Source: CAD feature listing. Evaluate the final solid. Frame: model axes, mm. Face numbers are marked on the shaded views. A direction names the side the tool comes from. Give positions to 0.01 mm unless a question says otherwise; leave off trailing zeros. Order: outer loops, then holes, each group sorted by start corner. A loop starts at its lowest first (then second) coordinate and runs counter-clockwise, first axis right, second up. Notation, with made-up numbers: M 37,-27 L 57,-27 A24 ccw 57,1 Z; hole C -12.75,-10.75 d11. An arc over 180 degrees is marked long. Return JSON: item names as keys, results as strings.
from build123d import *

# Parameters (mm, degrees)
F0_R     = 21
F1_DEPTH = 2
F2_R     = 19.1
F3_DEPTH = 8
F4_R     = 15.5
F5_DEPTH = 10
F6_R     = 1
F7_DEPTH = 8


with BuildPart() as f1:
    # F0 (on Top) → F1 (new body)
    with BuildSketch(Plane.XY):
        Circle(F0_R)
    extrude(amount=F1_DEPTH)

    # F2 (on face) → F3 (join)
    with BuildSketch(Plane.XY.offset(2)):
        Circle(F2_R)
    extrude(amount=F3_DEPTH)

    # F4 (on face) → F5 (cut, through all)
    with BuildSketch(Plane(origin=(0, 0, 0), x_dir=(1, 0, 0), z_dir=(0, 0, -1))):
        Circle(F4_R)
    extrude(amount=-F5_DEPTH, mode=Mode.SUBTRACT)

    # F6 (on face) → F7 (cut)
    with BuildSketch(Plane.XY.offset(10)):
        with Locations((-12.232947, 12.232947)):
            Circle(F6_R)
        with Locations((12.232947, 12.232947)):
            Circle(F6_R)
        with Locations((-12.232947, -12.232947)):
            Circle(F6_R)
        with Locations((12.232947, -12.232947)):
            Circle(F6_R)
    extrude(amount=-F7_DEPTH, mode=Mode.SUBTRACT)


solid = f1.part
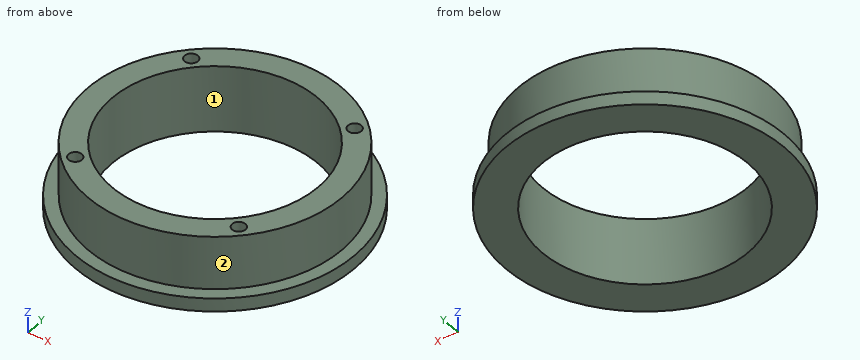
1. Section query C-C (z = 7). Return loops of the section in (x, y), then the cut area to 3 significant figures.
Evaluation:
{"outline": "C 0,0 d38.2; hole C 0,0 d31; hole C -12.23,-12.23 d2; hole C -12.23,12.23 d2; hole C 12.23,-12.23 d2; hole C 12.23,12.23 d2", "area": "379 mm^2"}
2. Section query D-D (x = 18.5). Return loops of the section in (y, z).
Evaluation:
{"outline": "M -9.94,0 L 9.94,0 L 9.94,2 L 4.75,2 L 4.75,10 L -4.75,10 L -4.75,2 L -9.94,2 Z"}
3. Ray query, probe 1 along Y at (x, z) = (-11.5, 8); probe 2 along Y at (x, z) = (0, 3.25). Return the intervals inside material, ascending.
Evaluation:
{"probe 1": "y = -15.25 to -12.91, -11.55 to -10.39, 10.39 to 11.55, 12.91 to 15.25", "probe 2": "y = -19.1 to -15.5, 15.5 to 19.1"}
4. Section query A-A (x = 0). Return loops of the section in (y, z), then the cut area to 3 significant figures.
Evaluation:
{"outline": "M -21,0 L -15.5,0 L -15.5,10 L -19.1,10 L -19.1,2 L -21,2 Z; M 15.5,0 L 21,0 L 21,2 L 19.1,2 L 19.1,10 L 15.5,10 Z", "area": "79.6 mm^2"}
5. First-contact query: pin 1 (1 mm diameter, centred on x = -12, y = -12.5, fed in from +Z); pin 2 (4 mm diameter, centred on y = -6, z = 3.5, fed in from +X); pin 3 (1 mm diameter, centred on x = -15.5, z = 4.5, fed in from +Y). Flat tips, straight axial feed; report the tip coordinate or a pass-through.
Evaluation:
{"pin 1": "stops at z = 2", "pin 2": "stops at x = 20.47", "pin 3": "stops at y = 11.82"}
6. Set-up query: the marked faces 1 and 2. Return all of +Z, -Z, +X, -X, +Y, -Y with unobstructed straight access to the full face (end or side cutting, diameter ignored); none if empty.
Evaluation:
{"face 1": "+Z, -Z", "face 2": "+Z"}
